Verification items for this drawing (mm, ordinates from the low corner). Coordinates: 2 decimals unless noted, no trailing zeros. Order: outer loops, then holes, each group sorted by start corner. A loop starts at its lowest first (then second) coordinate and runs counter-clockwise, first axis right, second up. Notation, with made-up numbers: (24, 24) -> (68, 24) arc R29 ccw to (68, 50) -> close; hole circle Ø10 at (-35, 9.5). An arc over 180 degrees is marked (long way). Write each question's results on one line, items separated by ' | '. Start each with the question number.
(1) Cross-section at A-A on y = 76.2. Enter the section's corners in (x, z) (1 decimal), and give its area (3 significant figures).
(2) Draft check along X on the marked faces 1, 2, 3 and 4. Enter one of: +X half, -X half, draft (parallel to the pull), parting line (faces both ways), or undercut.
(3) Go/stop test with a flat-tipped pin: pin 1 (7 mm diameter, centred on x = 8.03, y = 110.85, fed in from +Z). Record where the tip stops, or that it passes through.
(4) Cross-section at C-C on z = 1.5. Give the number of separate pieces and of enclosed holes in the cut face, and give its area (3 significant figures).
(5) Cross-section at D-D on x = 25. Enter the section's corners in (y, z) (1 decimal), and give its area (3 significant figures).
(6) Thickness scan on probe 1 along Y at (x, z) = (80.5, 7) (1 decimal); probe 2 along Y at (x, z) = (43, 9.75); probe 3 along Y at (x, z) = (81, 13.25) (1 decimal). Record the ranges inside material, lowest first. Write a range as [from, to].
(7) Cross-section at B-B on x = 75. Enter the section's corners in (y, z) (1 decimal).
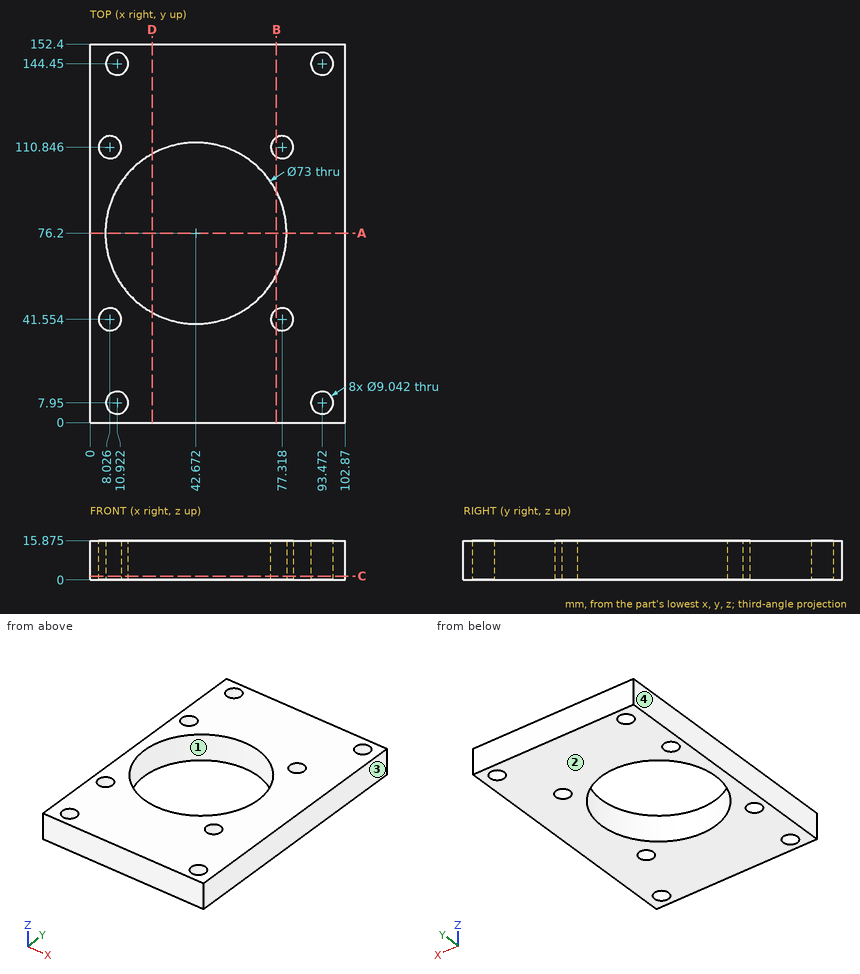
Results are:
1) outline: (0, 0) -> (6.2, 0) -> (6.2, 15.9) -> (0, 15.9) -> close; (79.2, 0) -> (102.9, 0) -> (102.9, 15.9) -> (79.2, 15.9) -> close | area: 474 mm2
2) face 1: undercut | face 2: draft | face 3: +X half | face 4: -X half
3) pin 1: passes through
4) separate pieces: 1 | enclosed holes: 9 | area: 11,000 mm2
5) outline: (0, 0) -> (44.3, 0) -> (44.3, 15.9) -> (0, 15.9) -> close; (108.1, 0) -> (152.4, 0) -> (152.4, 15.9) -> (108.1, 15.9) -> close | area: 1,410 mm2
6) probe 1: y = [0, 38.3], [44.8, 107.6], [114.1, 152.4] | probe 2: y = [0, 39.7], [112.7, 152.4] | probe 3: y = [0, 38.9], [44.2, 108.2], [113.5, 152.4]
7) outline: (0, 0) -> (37.7, 0) -> (37.7, 15.9) -> (0, 15.9) -> close; (45.4, 0) -> (59.3, 0) -> (59.3, 15.9) -> (45.4, 15.9) -> close; (93.1, 0) -> (107, 0) -> (107, 15.9) -> (93.1, 15.9) -> close; (114.7, 0) -> (152.4, 0) -> (152.4, 15.9) -> (114.7, 15.9) -> close
